Could you check a few things on this model? Use its own coordinates, in mm. Face numbers are marked on the shaded views. Coordinates: 2 decimals unless noted, no trailing zeros. Order: outer loops, then holes, each group sorted by start corner. A loop starts at its lowest first (then second) coordinate and runs counter-clockwise, first axis right, second up.
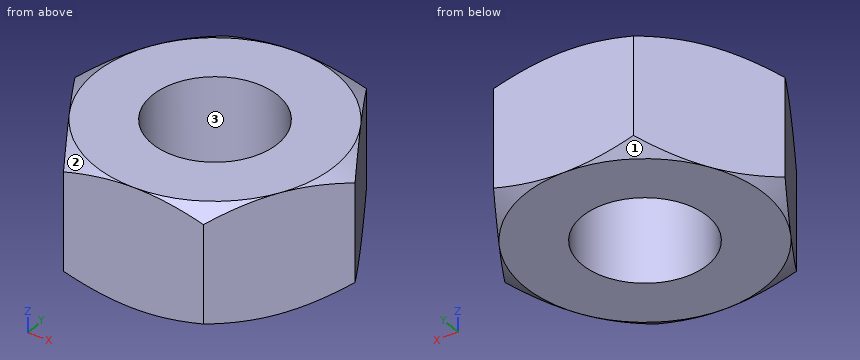
```python
from build123d import *

# Parameters (mm, degrees)
BOSS_EXTRUDE1_DEPTH = 6.5
M8_TAPPED_HOLE1_D   = 6.8


with BuildPart() as part:
    # Sketch1 → Boss-Extrude1 (new body)
    with BuildSketch(Plane.XY):
        Polygon((3.75277675, -6.5), (7.505553499, 0), (3.75277675, 6.5), (-3.75277675, 6.5), (-7.505553499, 0), (-3.75277675, -6.5), align=None)
    extrude(amount=BOSS_EXTRUDE1_DEPTH)

    # Sketch3 → Cut-Revolve1 (revolve, cut)
    with BuildSketch(Plane(origin=(0, 0, 0), x_dir=(0, 0, -1), z_dir=(1, 0, 0))):
        Polygon((-1.711637245, 9.464642673), (0, 6.5), (0, 9.464642673), align=None)
        Polygon((-6.5, 6.5), (-6.5, 9.37662807), (-4.839178009, 9.37662807), align=None)
    revolve(axis=Axis((0, 0, 0), (0, 0, -1)), mode=Mode.SUBTRACT)

    # M8 Tapped Hole1 (through all)
    with Locations(Plane.XY.offset(6.5)):
        with Locations((0, 0)):
            Hole(M8_TAPPED_HOLE1_D / 2)


solid = part.part
```
Item 1: I need wall thicknesses on line 1 (Y direction, x = 0, z = 1.75); line 2 (X direction, y = -0.75, z = 2.25); line 3 (X direction, y = -1.75, z = 3.5). Which ranges of each line are inside material? Lowest first, please.
Item 2: For pin 1 Ø1 at (y, z) = (-4, 2.5) entering from -X; pin 2 Ø5.5 at (x, y) = (0, 0) entering from -Z; pin 3 Ø2 at (y, z) = (4.5, 1) entering from +X, each with a flat end and sliding along its axis, tell me the tip position at first contact or that it passes through.
Item 3: Suppose I cut it at A-A (z = 2). List the corners of the cut face in (x, y) for me.
Item 4: Thinking about a two-plate mould opening in Y: for the marked faces 1, 2 and 3, which applies, +Y half, -Y half, draft (parallel to the pull), parting line (faces both ways), or undercut?
Geometry results:
1. line 1: y = -6.5 to -3.4, 3.4 to 6.5
1. line 2: x = -7.07 to -3.32, 3.32 to 7.07
1. line 3: x = -6.5 to -2.92, 2.92 to 6.5
2. pin 1: stops at x = -5.48
2. pin 2: passes through
2. pin 3: stops at x = 5.48
3. outline: (-7.51, 0) - (-3.75, -6.5) - (3.75, -6.5) - (7.51, 0) - (3.75, 6.5) - (-3.75, 6.5) - close; hole circle Ø6.8 at (0, 0)
4. face 1: +Y half
4. face 2: -Y half
4. face 3: undercut
